Source: CAD feature listing. Evaluate the final solid. Frame: model axes, mm. Round coordinates to 2 decimals unless told otherwise and drop trailing zeros. Loops run counter-clockwise (first coordinate to the right, second up) from the corner with the lowest first, then second, coordinate; pieces in that order, holes last. Notation, with made-up numbers: (-3.5, -33) -> (27.5, -33) arc R21 ccw to (27.5, -23) -> close; hole circle Ø7 at (3.25, -26). An arc over 180 degrees is marked (long way). Put each result on its own line as item: value. Start each with the question number.
1. Cut plane D-D (y = 2). Return the cut outline in (x, z).
2. Contact query for flat-ended pins moving along their axis: pin 1 (2 mm diameter, centred on x = -7.5, y = 3.5, fed in from +Z); pin 2 (11.5 mm diameter, centred on x = -50.02, z = -12.61, fed in from +Y); pin 3 (1 mm diameter, centred on x = -43.5, y = 1, fed in from -Z). Output: stop coordinate, or through.
3. Cut plane C-C (y = 7). Return the cut outline in (x, z), then the cut area to 3 significant figures.
4. Material intervals for L1, parallel to X at y = -3.25, z = -13; L2, parallel to X at y = 5.75, z = 5.5; L3, parallel to Z at x = 3, y = -1, sorted ascending.
5. Cut plane B-B (y = -1.25). Return the cut outline in (x, z), then the cut area to 3 significant figures.
6. Cut plane A-A (x = 2). Return the cut outline in (y, z).
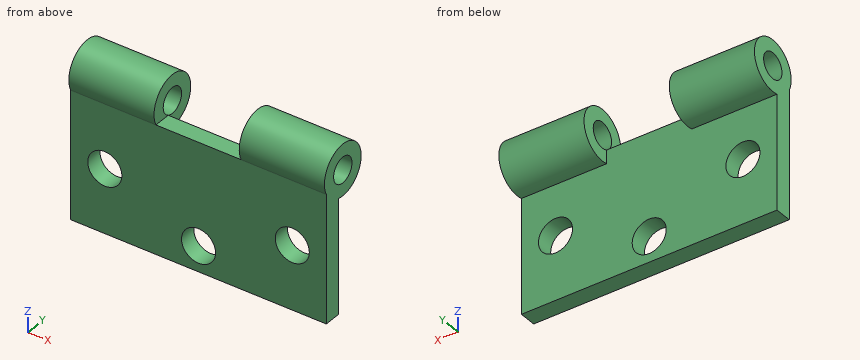
```python
from build123d import *

# Parameters (mm, degrees)
F0_W     = 76.2
F0_H     = 38.1
F1_DEPTH = 5.08
F2_R     = 7.62
F2_R_2   = 3.81
F3_DEPTH = 25.4
F4_R     = 7.62
F4_R_2   = 3.81
F5_DEPTH = 25.4
F6_R     = 5.08
F7_DEPTH = 5.08


# Not quite as in the source:
# - a feature names something its author has since deleted; it is built from what else it names


with BuildPart() as f1:
    # F0 (on Front) → F1 (new body)
    with BuildSketch(Plane.XZ):
        with Locations((-22.0833101058, -12.6055886477)):
            Rectangle(F0_W, F0_H)
    extrude(amount=F1_DEPTH)

    # F2 (on face) → F3 (join)
    with BuildSketch(Plane.YZ.offset(16.0166898942)):
        with Locations((1.74625, 9.8306645822)):
            Circle(F2_R)
        with Locations((1.74625, 9.8306645822)):
            Circle(F2_R_2, mode=Mode.SUBTRACT)
    extrude(amount=-F3_DEPTH)

    # F4 (on face) → F5 (join)
    with BuildSketch(Plane(origin=(-60.1833101058, 0, 0), x_dir=(0, -1, 0), z_dir=(-1, 0, 0))):
        with Locations((-1.74625, 9.8306645822)):
            Circle(F4_R)
        with Locations((-1.74625, 9.8306645822)):
            Circle(F4_R_2, mode=Mode.SUBTRACT)
    extrude(amount=-F5_DEPTH)

    # F6 (on face) → F7 (cut, through all)
    with BuildSketch(Plane.XZ.offset(5.08)):
        with Locations((-50.0233101058, -12.6055886477)):
            Circle(F6_R)
        with Locations((-22.0833101058, -24.0355886477)):
            Circle(F6_R)
        with Locations((5.8566898942, -12.6055886477)):
            Circle(F6_R)
    extrude(amount=-F7_DEPTH, mode=Mode.SUBTRACT)


solid = f1.part
```
Solution:
1. outline: (-60.18, 2.21) -> (-34.78, 2.21) -> (-34.78, 6.03) -> (-60.18, 6.03) -> close; (-60.18, 13.63) -> (-34.78, 13.63) -> (-34.78, 17.45) -> (-60.18, 17.45) -> close; (-9.38, 2.21) -> (16.02, 2.21) -> (16.02, 6.03) -> (-9.38, 6.03) -> close; (-9.38, 13.63) -> (16.02, 13.63) -> (16.02, 17.45) -> (-9.38, 17.45) -> close
2. pin 1: stops at z = 17.41
2. pin 2: stops at y = 0
2. pin 3: stops at z = 2.21
3. outline: (-60.18, 4.31) -> (-34.78, 4.31) -> (-34.78, 15.35) -> (-60.18, 15.35) -> close; (-9.38, 4.31) -> (16.02, 4.31) -> (16.02, 15.35) -> (-9.38, 15.35) -> close
3. area: 561 mm^2
4. L1: x = -60.18 to -55.09, -44.96 to 0.79, 10.92 to 16.02
4. L2: x = -60.18 to -34.78, -9.38 to 16.02
4. L3: z = -31.66 to -16.81, -8.4 to 7.19, 12.47 to 16.94
5. outline: (-60.18, -31.66) -> (16.02, -31.66) -> (16.02, 7.48) -> (-9.38, 7.48) -> (-9.38, 6.44) -> (-34.78, 6.44) -> (-34.78, 7.48) -> (-60.18, 7.48) -> close; (-60.18, 12.18) -> (-34.78, 12.18) -> (-34.78, 16.84) -> (-60.18, 16.84) -> close; (-9.38, 12.18) -> (16.02, 12.18) -> (16.02, 16.84) -> (-9.38, 16.84) -> close; hole circle Ø10.16 at (-50.02, -12.61); hole circle Ø10.16 at (-22.08, -24.04); hole circle Ø10.16 at (5.86, -12.61)
5. area: 2,950 mm^2
6. outline: (-5.08, -31.66) -> (0, -31.66) -> (0, -15.91) -> (-5.08, -15.91) -> close; (-5.08, -9.3) -> (0, -9.3) -> (0, 2.41) arc R7.62 ccw (long way) to (-5.08, 6.44) -> close; hole circle Ø7.62 at (1.75, 9.83)
